Verification items for the finished model (mm, model axes). A direction names the side the tool comes from. Coordinates: 2 decimals unless noted, no trailing zeros. Order: outer loops, then holes, each group sorted by start corner. A loop starts at its lowest first (then second) coordinate and runs counter-clockwise, first axis right, second up. Notation, with made-up numbers: (31, 19.25) - (50, 19.25) arc R19 cw to (50, 33.25) - close; hole circle Ø3 at (75, 58). An arc over 180 degrees is marked (long way). Answer as CSV lines item,"result". Start each with the question number.
1. Section check C-C (y = 3.55). Record the cut outline in (x, z), and give its area (3 significant figures).
2. Mould release check, pull along Z, two halves, no side actions. Record for faces 3 (the flat face through (18, 3, 0)), 4 (the cylindrical face through (1.856, 1.521, -2.42)), 5 (the cylindrical face through (4.48, 1.52, 2.33)): pulls with the +Z half, pulls with the -Z half, needs draft (parallel to the pull), parting line crosses it, or undercut.
3. Material ranges on L1, parallel to X at y = 3.5, z = 0; L2, parallel to X at y = 4.65, z = -0.5; L3, parallel to Z at x = 20, y = 4.2, recorded low to high. Write a range as [from, to].
4. Section check D-D (x = 14). Record the cut outline in (y, z).
5. Section check A-A (x = 20). Record the cut outline in (y, z), and give its area (3 significant figures).
6. Section check B-B (z = 0). Record the cut outline in (x, y), and give its area (3 significant figures).
7. Set-up check for faces 1 (the flat face through (0, 3, 0)), 2 (the flat face through (0, 4, -5.05)): record each of +Z, -Z, +X, -X, +Y, -Y from which the full face is reachable in a straight line by a thin tool's end or side.
8. Go/stop test with flat-tipped pins: pin 1 (3 mm diameter, centred on x = -21, z = 2, fed in from -Y); pin 2 (2 mm diameter, centred on x = -20, z = 0, fed in from +Y); pin 3 (2 mm diameter, centred on y = 1.5, z = -3, fed in from -X). Record where each tip stops, or that it passes through.
from build123d import *

# Parameters (mm, degrees)
SKETCH1_W           = 2
SKETCH1_H           = 3
SKETCH2_W           = 60
SKETCH2_H           = 10.1
BOSS_EXTRUDE1_DEPTH = 2
SKETCH3_R           = 1.25
CUT_EXTRUDE1_DEPTH  = 5


with BuildPart() as part:
    # Sketch1 → Revolve1 (revolve)
    with BuildSketch(Plane.XY, mode=Mode.PRIVATE) as revolve1_sk:
        with Locations((4.05, 1.5)):
            Rectangle(SKETCH1_W, SKETCH1_H)
    revolve(revolve1_sk.sketch.rotate(Axis((0, 97.022326023, 0), (0, -1, 0)), 90), axis=Axis((0, 97.022326023, 0), (0, -1, 0)))

    # Sketch2 → Boss-Extrude1 (add)
    with BuildSketch(Plane(origin=(0, 3, 0), x_dir=(1, 0, 0), z_dir=(0, 1, 0))):
        Rectangle(SKETCH2_W, SKETCH2_H)
    extrude(amount=BOSS_EXTRUDE1_DEPTH)

    # Sketch3 → Cut-Extrude1 (cut)
    with BuildSketch(Plane(origin=(0, 5, 0), x_dir=(1, 0, 0), z_dir=(0, 1, 0))):
        with Locations(Location((-20, 0, 0), (0, 0, 270))):
            Circle(SKETCH3_R)
        with Locations(Location((20, 0, 0), (0, 0, 90))):
            Circle(SKETCH3_R)
    extrude(amount=-CUT_EXTRUDE1_DEPTH, mode=Mode.SUBTRACT)


solid = part.part
Evaluation:
1,outline,"(-30, -5.05) - (30, -5.05) - (30, 5.05) - (-30, 5.05) - close; hole circle Ø2.5 at (-20, 0); hole circle Ø2.5 at (20, 0)"
1,area,"596 mm²"
2,face 3,"needs draft"
2,face 4,"undercut"
2,face 5,"parting line crosses it"
3,L1,"x = [-30, -21.25], [-18.75, 18.75], [21.25, 30]"
3,L2,"x = [-30, -21.15], [-18.85, 18.85], [21.15, 30]"
3,L3,"z = [-5.05, -1.25], [1.25, 5.05]"
4,outline,"(3, -5.05) - (5, -5.05) - (5, 5.05) - (3, 5.05) - close"
5,outline,"(3, -5.05) - (5, -5.05) - (5, -1.25) - (3, -1.25) - close; (3, 1.25) - (5, 1.25) - (5, 5.05) - (3, 5.05) - close"
5,area,"15.2 mm²"
6,outline,"(-30, 3) - (-21.25, 3) - (-21.25, 5) - (-30, 5) - close; (-18.75, 3) - (-5.05, 3) - (-5.05, 0) - (-3.05, 0) - (-3.05, 3) - (3.05, 3) - (3.05, 0) - (5.05, 0) - (5.05, 3) - (18.75, 3) - (18.75, 5) - (-18.75, 5) - close; (21.25, 3) - (30, 3) - (30, 5) - (21.25, 5) - close"
6,area,"122 mm²"
7,face 1,"-Y"
7,face 2,"-Z, +X, -X, +Y, -Y"
8,pin 1,"stops at y = 3"
8,pin 2,"passes through"
8,pin 3,"stops at x = -4.64"
